from build123d import *

# Parameters (mm, degrees)
SKETCH1_W           = 40.64
SKETCH1_H           = 6.35
BOSS_EXTRUDE1_DEPTH = 8.89
SKETCH2_W           = 5.08
SKETCH2_H           = 8.89
BOSS_EXTRUDE2_DEPTH = 7.62
SKETCH3_W           = 5.08
SKETCH3_H           = 8.89
BOSS_EXTRUDE3_DEPTH = 7.62
SKETCH4_W           = 3.556
SKETCH4_H           = 3.556
CUT_EXTRUDE1_DEPTH  = 2.54
BOSS_EXTRUDE4_DEPTH = 2.54
SKETCH6_W           = 40.64
SKETCH6_H           = 3.683
BOSS_EXTRUDE5_DEPTH = 2.54
SKETCH7_W           = 3.556
SKETCH7_H           = 4.572
CUT_EXTRUDE2_DEPTH  = 2.54
BOSS_EXTRUDE6_START = 2.54
BOSS_EXTRUDE6_DEPTH = 2.54
WRAP2_SECTION_W     = 0.762
WRAP2_SECTION_H     = 1.016
WRAP2_ANGLE         = 76.394372684
SKETCH11_W          = 0.508
SKETCH11_H          = 6.35
CUT_EXTRUDE3_DEPTH  = 1.27
SKETCH12_W          = 2.032
SKETCH12_H          = 2.032
BOSS_EXTRUDE7_DEPTH = 2.032


with BuildPart() as part:
    # Sketch1 → Boss-Extrude1 (new body)
    with BuildSketch(Plane.XY):
        with Locations((20.32, 3.175)):
            Rectangle(SKETCH1_W, SKETCH1_H)
    extrude(amount=BOSS_EXTRUDE1_DEPTH)

    # Sketch2 → Boss-Extrude2 (add)
    with BuildSketch(Plane(origin=(0, 6.35, 0), x_dir=(1, 0, 0), z_dir=(0, 1, 0))):
        with Locations((2.54, -4.445)):
            Rectangle(SKETCH2_W, SKETCH2_H)
    extrude(amount=BOSS_EXTRUDE2_DEPTH)

    # Sketch3 → Boss-Extrude3 (add)
    with BuildSketch(Plane(origin=(0, 6.35, 0), x_dir=(1, 0, 0), z_dir=(0, 1, 0))):
        with Locations((38.1, -4.445)):
            Rectangle(SKETCH3_W, SKETCH3_H)
    extrude(amount=BOSS_EXTRUDE3_DEPTH)

    # Sketch4 → Cut-Extrude1 (cut)
    with BuildSketch(Plane(origin=(5.08, 0, 0), x_dir=(0, 0, -1), z_dir=(1, 0, 0))):
        with Locations((-1.778, 12.192)):
            Rectangle(SKETCH4_W, SKETCH4_H)
    extrude(amount=-CUT_EXTRUDE1_DEPTH, mode=Mode.SUBTRACT)

    # Sketch5 → Boss-Extrude4 (add)
    with BuildSketch(Plane.ZY):
        with BuildLine():
            Line((8.255, 13.97), (0.635, 13.97))
            ThreePointArc((0.635, 13.97), (4.445, 10.16), (8.255, 13.97))
        make_face()
    extrude(amount=BOSS_EXTRUDE4_DEPTH)

    # Sketch6 → Boss-Extrude5 (add)
    with BuildSketch(Plane(origin=(0, 0, 0), x_dir=(-1, 0, 0), z_dir=(0, 0, -1))):
        with Locations((-20.32, 1.8415)):
            Rectangle(SKETCH6_W, SKETCH6_H)
    extrude(amount=BOSS_EXTRUDE5_DEPTH)

    # Sketch7 → Cut-Extrude2 (cut)
    with BuildSketch(Plane.ZY.offset(-35.56)):
        with Locations((1.778, 11.684)):
            Rectangle(SKETCH7_W, SKETCH7_H)
    extrude(amount=-CUT_EXTRUDE2_DEPTH, mode=Mode.SUBTRACT)

    # Sketch8 → Boss-Extrude6 (add)
    with BuildSketch(Plane(origin=(40.64, 0, 0), x_dir=(0, 0, -1), z_dir=(1, 0, 0)).offset(BOSS_EXTRUDE6_START)):
        with BuildLine():
            Line((-0.635, 13.97), (-8.255, 13.97))
            ThreePointArc((-8.255, 13.97), (-4.445, 10.16), (-0.635, 13.97))
        make_face()
    extrude(amount=-BOSS_EXTRUDE6_DEPTH)

    # Wrap2 section (on wrap section) → Wrap2 (revolve)
    with BuildSketch(Plane(origin=(0, 13.97, 4.445), x_dir=(0, -0.8032608103480625, 0.5956274595407551), z_dir=(0, 0.5956274595407551, 0.8032608103480625))):
        with Locations((4.191, -1.397)):
            Rectangle(WRAP2_SECTION_W, WRAP2_SECTION_H)
    revolve(axis=Axis((0, 13.97, 4.445), (1, 0, 0)), revolution_arc=WRAP2_ANGLE)

    # Sketch11 → Cut-Extrude3 (cut)
    with BuildSketch(Plane.XZ):
        with Locations((20.32, 0.635)):
            Rectangle(SKETCH11_W, SKETCH11_H)
    extrude(amount=-CUT_EXTRUDE3_DEPTH, mode=Mode.SUBTRACT)

    # Sketch12 → Boss-Extrude7 (add)
    with BuildSketch(Plane(origin=(0, 13.97, 0), x_dir=(1, 0, 0), z_dir=(0, 1, 0))):
        with Locations((40.64, -4.445)):
            Rectangle(SKETCH12_W, SKETCH12_H)
    extrude(amount=BOSS_EXTRUDE7_DEPTH)


solid = part.part
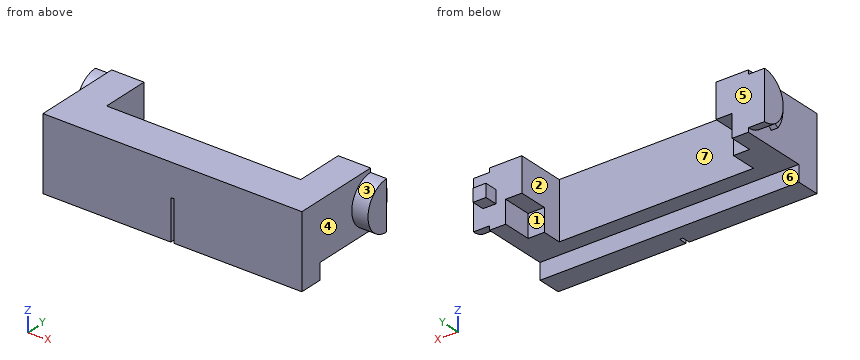
Read the model definition and answer for the solid it produces. Units are mm, in the model's axes. Face numbers are marked on the shaded views. A direction names the side the tool comes from. Coordinates: 2 decimals unless noted, no trailing zeros. Loops run counter-clockwise (first coordinate to the right, second up) from the corner with the lowest first, then second, coordinate; pieces in that order, holes last.
Q1. The part is cut by section A-A on x = 10. Write down the section's boundary in (y, z).
Q2. The part is cut by section C-C on y = 4.5. Write down the section's boundary in (x, z).
Q3. Which of the six approach directions +Z, -Z, +X, -X, +Y, -Y give full straight-line access (tool end or side, diameter ignored) to the marked faces 5, 6 and 7?
Q4. Consider probe 1 along X at (y, z) = (10.25, 4.5); probe 2 along X at (y, z) = (12, 1); probe 3 along Z at (x, y) = (14, 5.25). Determine where each line is inside the solid, lowest interval first.
Q5. Each of these flat-tipped pins is pushed along its axis until it touches: pin 1 Ø0.6 at (y, z) = (0.5, 1) entering from +X; pin 2 Ø1.5 at (x, z) = (7.5, 4) entering from +Y; pin 3 Ø1 at (y, z) = (3.5, 0.5) entering from -X. Where does it stop, or does it pass through?
Q6. The part is cut by section D-D on x = 2. Write down the section's boundary in (y, z), and give its area (3 significant figures).
Q7. The mould has two halves that part along X. Classify the marked faces 1, 2, 3 and 4: +X half, -X half, draft (parallel to the pull), parting line (faces both ways), or undercut.
Q8. The part is cut by section B-B on z = 7.75. Write down the section's boundary in (x, y).
Results below:
1. outline: (0, -2.54) - (3.68, -2.54) - (3.68, 0) - (6.35, 0) - (6.35, 8.89) - (0, 8.89) - close
2. outline: (0, 0) - (40.64, 0) - (40.64, 8.89) - (0, 8.89) - close
3. face 5: +Z, -Z, -X, +Y
3. face 6: -Z, +X, -X, +Y
3. face 7: +Z, -Z, +Y
4. probe 1: x = -2.54 to 5.08, 35.56 to 43.18
4. probe 2: x = 0 to 2.54, 38.1 to 40.64
4. probe 3: z = 0 to 8.89
5. pin 1: stops at x = 40.64
5. pin 2: stops at y = 6.35
5. pin 3: stops at x = 0
6. outline: (0, -2.54) - (3.68, -2.54) - (3.68, 0) - (13.97, 0) - (13.97, 8.89) - (0, 8.89) - close
6. area: 134 mm2
7. face 1: undercut
7. face 2: undercut
7. face 3: draft
7. face 4: +X half
8. outline: (-2.54, 12.07) - (0, 12.07) - (0, 0) - (40.64, 0) - (40.64, 12.07) - (43.18, 12.07) - (43.18, 13.97) - (35.56, 13.97) - (35.56, 6.35) - (5.08, 6.35) - (5.08, 13.97) - (-2.54, 13.97) - close
